For this review, take the finished solid that the model builds, in its own axes (mm). Face numbers are marked on the shaded views. A direction names the side the tool comes from. Give positions to 0.01 mm unless a question says otherwise; leave off trailing zeros. Loops run counter-clockwise (first coordinate to the right, second up) from the corner with the lowest first, then second, coordinate; pieces in that order, holes last. Notation, with made-up numbers: (-32.5, -17) - (8.5, -17) arc R32 ccw to (8.5, 9) - close; hole circle Ø10 at (50, 43.5). An arc over 180 degrees is marked (long way). Use CSV: the item, a comma, the result in double quotes. Start each with the question number.
1. Wall thickness on line 1 (Y direction, x = -7.25, z = -16.5); line 2 (X direction, y = 19.5, z = 8.5); line 3 (Z direction, x = -2.25, y = 11): over which ranges is each line inside the solid? List them lowest first.
2. Take a section at B-B on y = 16. Give the boundary of the cut face in (x, z), plus the area to 3 significant figures.
3. Mouldability with a two-part tool opening along X and no side actions: class the marked faces 3, 4 and 5 as pulls with the +X half, pulls with the -X half, needs draft (parallel to the pull), parting line crosses it, or undercut.
4. For pin 1 (1 mm diameter, centred on y = 28.5, z = 14, fed in from +X); pin 2 (8 mm diameter, centred on x = -7, z = 5, fed in from +Y); pin 3 (11 mm diameter, centred on x = 4.5, z = -11.5, fed in from +Y); pin 4 (12 mm diameter, centred on x = -8.5, z = 7, fed in from -Y), all flat-tipped, find the tip position at first contact; note any pin that passes through.
5. For the marked faces 1 and 2, list the 3-axis set-ups (+Z, -Z, +X, -X, +Y, -Y) from which the entire face can be reached by the end or side of a thin tool; tool diameter is ignored.
6. Take a section at C-C on z = -6.5. Give the boundary of the cut face in (x, y).
7. Take a section at A-A on x = 0. Give the boundary of the cut face in (y, z).
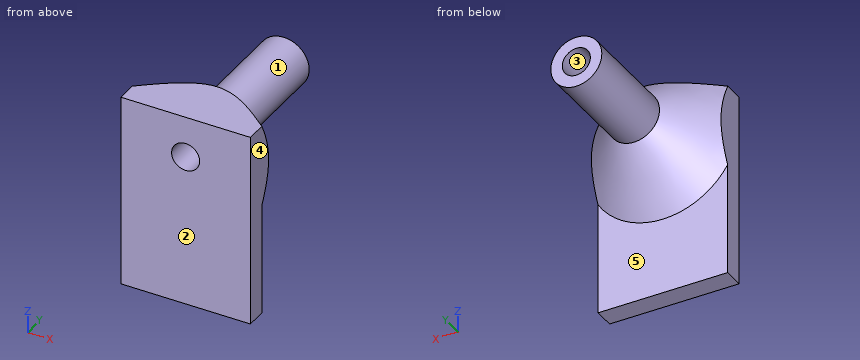
```python
from build123d import *

# Parameters (mm, degrees)
SKETCH1_W           = 25.4
SKETCH1_H           = 38.1
BOSS_EXTRUDE1_DEPTH = 4
SKETCH2_R           = 5
BOSS_EXTRUDE2_DEPTH = 30
SKETCH3_R           = 2.75
CUT_EXTRUDE1_DEPTH  = 40
CHAMFER1_SIZE       = 10


with BuildPart() as part:
    # Sketch1 → Boss-Extrude1 (new body)
    with BuildSketch(Plane(origin=(0, 0, 0), x_dir=(1, 0, 0), z_dir=(0, 1, 0))):
        Rectangle(SKETCH1_W, SKETCH1_H)
    extrude(amount=BOSS_EXTRUDE1_DEPTH)

    # Sketch2 → Boss-Extrude2 (add)
    with BuildSketch(Plane(origin=(0, 4, 0), x_dir=(1, 0, 0), z_dir=(0, 1, 0))):
        with Locations(Location((0, -10.9531854, 0), (0, 0, 270))):
            Circle(SKETCH2_R)
    extrude(amount=BOSS_EXTRUDE2_DEPTH)

    # Sketch3 → Cut-Extrude1 (cut)
    with BuildSketch(Plane(origin=(0, 34, 0), x_dir=(1, 0, 0), z_dir=(0, 1, 0))):
        with Locations(Location((0, -10.9531854, 0), (0, 0, 270))):
            Circle(SKETCH3_R)
    extrude(amount=-CUT_EXTRUDE1_DEPTH, mode=Mode.SUBTRACT)

    # Chamfer1
    # the kernel refuses this chamfer: 10 mm, written as the material it adds along each edge
    with BuildSketch(Plane(origin=(0, 4, 10.9531854), x_dir=(0, 0, 1), z_dir=(-1, 0, 0))) as chamfer1_piece_1_section:
        Polygon((5 + CHAMFER1_SIZE, 0), (5, CHAMFER1_SIZE), (5, 0), align=None)
    chamfer1_piece_1 = revolve(axis=Axis((0, 4, 10.9531854), (0, 1, 0)), mode=Mode.PRIVATE)
    chamfer1_piece_1 = split(chamfer1_piece_1, bisect_by=Plane(origin=(-12.7, 8.904804992, 1.048380408), z_dir=(1, 0, 0)), keep=Keep.TOP, mode=Mode.PRIVATE)
    chamfer1_piece_1 = split(chamfer1_piece_1, bisect_by=Plane(origin=(12.7, 8.904804992, 1.048380408), z_dir=(-1, 0, 0)), keep=Keep.TOP, mode=Mode.PRIVATE)
    chamfer1_piece_1 = split(chamfer1_piece_1, bisect_by=Plane(origin=(0, 8.904804992, 19.05), z_dir=(0, 0, -1)), keep=Keep.TOP, mode=Mode.PRIVATE)
    add(chamfer1_piece_1)


solid = part.part
```
Check result:
1,line 1,"y = 0 to 4"
1,line 2,"x = -4.36 to -1.24, 1.24 to 4.36"
1,line 3,"z = 3.28 to 9.37, 12.53 to 18.63"
2,outline,"circle Ø10 at (0, 10.95); hole circle Ø5.5 at (0, 10.95)"
2,area,"54.8 mm²"
3,face 3,"undercut"
3,face 4,"pulls with the +X half"
3,face 5,"needs draft"
4,pin 1,"stops at x = 4.3"
4,pin 2,"stops at y = 13.81"
4,pin 3,"stops at y = 4"
4,pin 4,"stops at y = 0"
5,face 1,"+Y"
5,face 2,"+Z, -Z, +X, -X, -Y"
6,outline,"(-12.7, 0) - (12.7, 0) - (12.7, 4) - (-12.7, 4) - close"
7,outline,"(0, -19.05) - (4, -19.05) - (4, -4.05) - (14, 5.95) - (34, 5.95) - (34, 8.2) - (0, 8.2) - close; (0, 13.7) - (34, 13.7) - (34, 15.95) - (14, 15.95) - (10.9, 19.05) - (0, 19.05) - close"
